Design review of the part shown in the three views and the two pictorial views. Dimensions are in mm from the part's minimum x, y and z. Round coordinates to 2 decimals unless told otherwise and drop trailing zeros. Loops run counter-clockwise (first coordinate to the right, second up) from the corner with the lowest first, then second, coordinate; pieces in that order, holes last.
1. Consider section B-B on z = 3. State the section outline as (x, y) points.
2. Consider section A-A on x = 3. State the section outline as (y, z) points.
3. Consider section D-D on x = 125. State the section outline as (y, z) points.
4. Consider section C-C on z = 40. State the section outline as (x, y) points, then the cut area to 3 significant figures.
5. Clearance check with a flat-ended pin moving along its axis: pin 1 Ø2.5 at (x, z) = (162, 3) entering from -Y. State where the tip first meets the part, or that it passes through.
6. To check wall thickness, follow line 1 along Z through (x, y) = (162, 42); line 2 along X through (y, z) = (42.2, 3); line 3 along Y through (x, z) = (94.5, 64). State the ranges of each line that lie inside material, in increasing order.
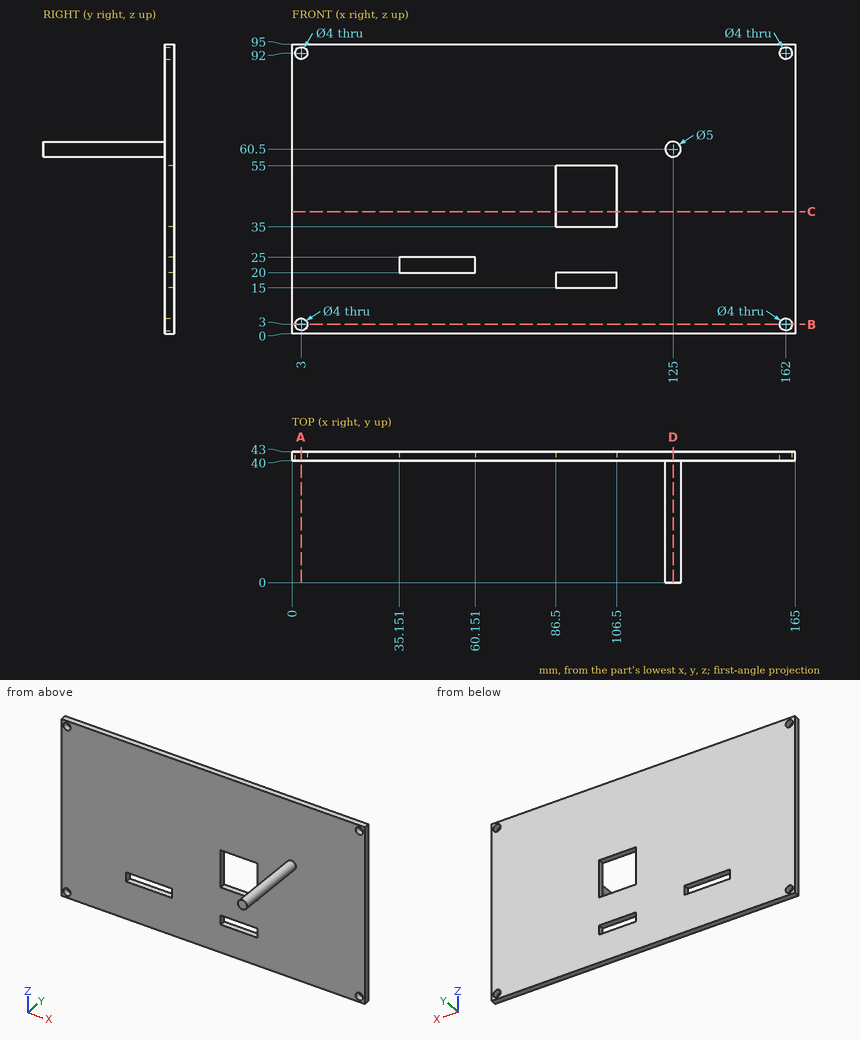
Resolved:
1. outline: (0, 40) - (1, 40) - (1, 43) - (0, 43) - close; (5, 40) - (160, 40) - (160, 43) - (5, 43) - close; (164, 40) - (165, 40) - (165, 43) - (164, 43) - close
2. outline: (40, 0) - (43, 0) - (43, 1) - (40, 1) - close; (40, 5) - (43, 5) - (43, 90) - (40, 90) - close; (40, 94) - (43, 94) - (43, 95) - (40, 95) - close
3. outline: (0, 58) - (40, 58) - (40, 0) - (43, 0) - (43, 95) - (40, 95) - (40, 63) - (0, 63) - close
4. outline: (0, 40) - (86.5, 40) - (86.5, 43) - (0, 43) - close; (106.5, 40) - (165, 40) - (165, 43) - (106.5, 43) - close
4. area: 435 mm2
5. pin 1: passes through
6. line 1: z = 0 to 1, 5 to 90, 94 to 95
6. line 2: x = 0 to 1, 5 to 160, 164 to 165
6. line 3: y = 40 to 43
